Here's how the part is built. I have some questions about the finished solid (model axes, mm). Face numbers are marked on the shaded views. A direction names the side the tool comes from. Coordinates: 2 decimals unless noted, no trailing zeros. Order: outer loops, then holes, each group sorted by start corner. A loop starts at its lowest first (then second) coordinate and runs counter-clockwise, first axis right, second up. Notation, with made-up numbers: (12, 71) - (63, 71) arc R28 ccw to (63, 94) - close; hole circle Ø11 at (28, 27.25). An arc over 180 degrees is marked (long way). Answer in a Markdown table with one row per item. Add a question column.
Item 1: Will these pins go through, and if not, where does the flat tip stop? pin 1 Ø1 at (x, z) = (1, 1) entering from +Y; pin 2 Ø12 at (x, y) = (0, 0) entering from -Z; pin 3 Ø1.5 at (x, z) = (13, 4.5) entering from -Y; pin 4 Ø3 at (x, z) = (12.5, 4) entering from +Y.
Item 2: If I drill on line 1 along Y through (x, z) = (0, 3.5); line 2 along X through (y, z) = (-31, 0.5); line 3 along Y through (x, z) = (-35, 4.2), over which ranges is the centre line in solid material (lowest first)? Write a range as from..to.
Item 3: I want a section at C-C (x = -27.5). Please give me the cut outline in (y, z), plus the area to 3 significant figures.
Item 4: I want a section at A-A (x = 0). Please give me the cut outline in (y, z), plus the area to 3 significant figures.
Item 5: Thinking about a two-plate mould opening in Y: for the marked faces 1, 2, 3 and 4, which applies, +Y half, -Y half, draft (parallel to the pull), parting line (faces both ways), or undercut?
Item 6: I want a section at D-D (y = 12). Please give me the cut outline in (x, z).
Item 7: On a 3-axis mill with a long thin cutter (end or side, diameter ignored), from which of +Z, -Z, +X, -X, +Y, -Y can I reach the whole of each face in a straight line? I mean the marked faces 5, 6, 7 and 8. Say none if no direction works.
```python
from build123d import *

# Parameters (mm, degrees)
SKETCH1_R           = 40
SKETCH1_R_2         = 10
BOSS_EXTRUDE1_DEPTH = 6
CUT_EXTRUDE1_START  = -6
CUT_EXTRUDE1_DEPTH  = 6
CIRPATTERN1_DEPTH   = 6


# Read off the part's stored shape, not the designer's step: CirPattern1
with BuildPart() as part:
    # Sketch1 → Boss-Extrude1 (new body)
    with BuildSketch(Plane.XY):
        Circle(SKETCH1_R)
        Circle(SKETCH1_R_2, mode=Mode.SUBTRACT)
    extrude(amount=BOSS_EXTRUDE1_DEPTH)

    # Sketch2 → Cut-Extrude1 (cut)
    with BuildSketch(Plane.XY.offset(6).offset(CUT_EXTRUDE1_START)):
        with BuildLine():
            Line((-3.601715358, 39.837515566), (-1.869030862, 35.288154767))
            ThreePointArc((-1.869030862, 35.288154767), (0, 34), (1.869030862, 35.288154767))
            Line((1.869030862, 35.288154767), (3.601715358, 39.837515566))
            ThreePointArc((3.601715358, 39.837515566), (0, 40), (-3.601715358, 39.837515566))
        make_face()
    extrude(amount=CUT_EXTRUDE1_DEPTH, mode=Mode.SUBTRACT)

    # CirPattern1 outline → CirPattern1 (cut)
    with BuildSketch(Plane.XY):
        with BuildLine():
            Line((-13.789697621, 37.547892611), (-10.9385917, 33.601999269))
            ThreePointArc((-10.9385917, 33.601999269), (-8.799847533, 32.841478094), (-7.32790134, 34.569480835))
            Line((-7.32790134, 34.569480835), (-6.831717855, 39.41227767))
            ThreePointArc((-6.831717855, 39.41227767), (-10.352761804, 38.637033051), (-13.789697621, 37.547892611))
        make_face()
        with BuildLine():
            Line((10.9385917, 33.601999269), (13.789697621, 37.547892611))
            ThreePointArc((13.789697621, 37.547892611), (10.352761804, 38.637033051), (6.831717855, 39.41227767))
            Line((6.831717855, 39.41227767), (7.32790134, 34.569480835))
            ThreePointArc((7.32790134, 34.569480835), (8.799847533, 32.841478094), (10.9385917, 33.601999269))
        make_face()
        with BuildLine():
            Line((19.262705591, 29.62592305), (23.03793478, 32.699442825))
            ThreePointArc((23.03793478, 32.699442825), (20, 34.641016151), (16.799580786, 36.301158183))
            Line((16.799580786, 36.301158183), (16.025449176, 31.494953912))
            ThreePointArc((16.025449176, 31.494953912), (17, 29.444863729), (19.262705591, 29.62592305))
        make_face()
        with BuildLine():
            Line((26.274097929, 23.630889134), (30.716174756, 25.622580049))
            ThreePointArc((30.716174756, 25.622580049), (28.284271247, 28.284271247), (25.622580049, 30.716174756))
            Line((25.622580049, 30.716174756), (23.630889134, 26.274097929))
            ThreePointArc((23.630889134, 26.274097929), (24.04163056, 24.04163056), (26.274097929, 23.630889134))
        make_face()
        with BuildLine():
            Line((31.494953912, 16.025449176), (36.301158183, 16.799580786))
            ThreePointArc((36.301158183, 16.799580786), (34.641016151, 20), (32.699442825, 23.03793478))
            Line((32.699442825, 23.03793478), (29.62592305, 19.262705591))
            ThreePointArc((29.62592305, 19.262705591), (29.444863729, 17), (31.494953912, 16.025449176))
        make_face()
        with BuildLine():
            Line((34.569480835, 7.32790134), (39.41227767, 6.831717855))
            ThreePointArc((39.41227767, 6.831717855), (38.637033052, 10.352761804), (37.547892611, 13.789697621))
            Line((37.547892611, 13.789697621), (33.601999269, 10.9385917))
            ThreePointArc((33.601999269, 10.9385917), (32.841478094, 8.799847533), (34.569480835, 7.32790134))
        make_face()
        with BuildLine():
            Line((35.288154767, -1.869030862), (39.837515566, -3.601715358))
            ThreePointArc((39.837515566, -3.601715358), (40, 0), (39.837515566, 3.601715358))
            Line((39.837515566, 3.601715358), (35.288154767, 1.869030862))
            ThreePointArc((35.288154767, 1.869030862), (34, 0), (35.288154767, -1.869030862))
        make_face()
        with BuildLine():
            Line((33.601999269, -10.9385917), (37.547892611, -13.789697621))
            ThreePointArc((37.547892611, -13.789697621), (38.637033052, -10.352761804), (39.41227767, -6.831717855))
            Line((39.41227767, -6.831717855), (34.569480835, -7.32790134))
            ThreePointArc((34.569480835, -7.32790134), (32.841478094, -8.799847533), (33.601999269, -10.9385917))
        make_face()
        with BuildLine():
            Line((29.62592305, -19.262705591), (32.699442825, -23.03793478))
            ThreePointArc((32.699442825, -23.03793478), (34.641016151, -20), (36.301158183, -16.799580786))
            Line((36.301158183, -16.799580786), (31.494953912, -16.025449176))
            ThreePointArc((31.494953912, -16.025449176), (29.444863729, -17), (29.62592305, -19.262705591))
        make_face()
        with BuildLine():
            Line((23.630889134, -26.274097929), (25.622580049, -30.716174756))
            ThreePointArc((25.622580049, -30.716174756), (28.284271247, -28.284271247), (30.716174756, -25.622580049))
            Line((30.716174756, -25.622580049), (26.274097929, -23.630889134))
            ThreePointArc((26.274097929, -23.630889134), (24.04163056, -24.04163056), (23.630889134, -26.274097929))
        make_face()
        with BuildLine():
            Line((16.025449176, -31.494953912), (16.799580786, -36.301158183))
            ThreePointArc((16.799580786, -36.301158183), (20, -34.641016151), (23.03793478, -32.699442825))
            Line((23.03793478, -32.699442825), (19.262705591, -29.62592305))
            ThreePointArc((19.262705591, -29.62592305), (17, -29.444863729), (16.025449176, -31.494953912))
        make_face()
        with BuildLine():
            Line((7.32790134, -34.569480835), (6.831717855, -39.41227767))
            ThreePointArc((6.831717855, -39.41227767), (10.352761804, -38.637033052), (13.789697621, -37.547892611))
            Line((13.789697621, -37.547892611), (10.9385917, -33.601999269))
            ThreePointArc((10.9385917, -33.601999269), (8.799847533, -32.841478094), (7.32790134, -34.569480835))
        make_face()
        with BuildLine():
            Line((-1.869030862, -35.288154767), (-3.601715358, -39.837515566))
            ThreePointArc((-3.601715358, -39.837515566), (0, -40), (3.601715358, -39.837515566))
            Line((3.601715358, -39.837515566), (1.869030862, -35.288154767))
            ThreePointArc((1.869030862, -35.288154767), (0, -34), (-1.869030862, -35.288154767))
        make_face()
        with BuildLine():
            Line((-10.9385917, -33.601999269), (-13.789697621, -37.547892611))
            ThreePointArc((-13.789697621, -37.547892611), (-10.352761804, -38.637033052), (-6.831717855, -39.41227767))
            Line((-6.831717855, -39.41227767), (-7.32790134, -34.569480835))
            ThreePointArc((-7.32790134, -34.569480835), (-8.799847533, -32.841478094), (-10.9385917, -33.601999269))
        make_face()
        with BuildLine():
            Line((-19.262705591, -29.62592305), (-23.03793478, -32.699442825))
            ThreePointArc((-23.03793478, -32.699442825), (-20, -34.641016151), (-16.799580786, -36.301158183))
            Line((-16.799580786, -36.301158183), (-16.025449176, -31.494953912))
            ThreePointArc((-16.025449176, -31.494953912), (-17, -29.444863729), (-19.262705591, -29.62592305))
        make_face()
        with BuildLine():
            Line((-26.274097929, -23.630889134), (-30.716174756, -25.622580049))
            ThreePointArc((-30.716174756, -25.622580049), (-28.284271247, -28.284271247), (-25.622580049, -30.716174756))
            Line((-25.622580049, -30.716174756), (-23.630889134, -26.274097929))
            ThreePointArc((-23.630889134, -26.274097929), (-24.04163056, -24.04163056), (-26.274097929, -23.630889134))
        make_face()
        with BuildLine():
            Line((-31.494953912, -16.025449176), (-36.301158183, -16.799580786))
            ThreePointArc((-36.301158183, -16.799580786), (-34.641016151, -20), (-32.699442825, -23.03793478))
            Line((-32.699442825, -23.03793478), (-29.62592305, -19.262705591))
            ThreePointArc((-29.62592305, -19.262705591), (-29.444863729, -17), (-31.494953912, -16.025449176))
        make_face()
        with BuildLine():
            Line((-34.569480835, -7.32790134), (-39.41227767, -6.831717855))
            ThreePointArc((-39.41227767, -6.831717855), (-38.637033052, -10.352761804), (-37.547892611, -13.789697621))
            Line((-37.547892611, -13.789697621), (-33.601999269, -10.9385917))
            ThreePointArc((-33.601999269, -10.9385917), (-32.841478094, -8.799847533), (-34.569480835, -7.32790134))
        make_face()
        with BuildLine():
            Line((-35.288154767, 1.869030862), (-39.837515566, 3.601715358))
            ThreePointArc((-39.837515566, 3.601715358), (-40, 0), (-39.837515566, -3.601715358))
            Line((-39.837515566, -3.601715358), (-35.288154767, -1.869030862))
            ThreePointArc((-35.288154767, -1.869030862), (-34, 0), (-35.288154767, 1.869030862))
        make_face()
        with BuildLine():
            Line((-33.601999269, 10.9385917), (-37.547892611, 13.789697621))
            ThreePointArc((-37.547892611, 13.789697621), (-38.637033052, 10.352761804), (-39.41227767, 6.831717855))
            Line((-39.41227767, 6.831717855), (-34.569480835, 7.32790134))
            ThreePointArc((-34.569480835, 7.32790134), (-32.841478094, 8.799847533), (-33.601999269, 10.9385917))
        make_face()
        with BuildLine():
            Line((-29.62592305, 19.262705591), (-32.699442825, 23.03793478))
            ThreePointArc((-32.699442825, 23.03793478), (-34.641016151, 20), (-36.301158183, 16.799580786))
            Line((-36.301158183, 16.799580786), (-31.494953912, 16.025449176))
            ThreePointArc((-31.494953912, 16.025449176), (-29.444863729, 17), (-29.62592305, 19.262705591))
        make_face()
        with BuildLine():
            Line((-23.630889134, 26.274097929), (-25.622580049, 30.716174756))
            ThreePointArc((-25.622580049, 30.716174756), (-28.284271247, 28.284271247), (-30.716174756, 25.622580049))
            Line((-30.716174756, 25.622580049), (-26.274097929, 23.630889134))
            ThreePointArc((-26.274097929, 23.630889134), (-24.04163056, 24.04163056), (-23.630889134, 26.274097929))
        make_face()
        with BuildLine():
            Line((-16.025449176, 31.494953912), (-16.799580786, 36.301158183))
            ThreePointArc((-16.799580786, 36.301158183), (-20, 34.641016151), (-23.03793478, 32.699442825))
            Line((-23.03793478, 32.699442825), (-19.262705591, 29.62592305))
            ThreePointArc((-19.262705591, 29.62592305), (-17, 29.444863729), (-16.025449176, 31.494953912))
        make_face()
    extrude(amount=CIRPATTERN1_DEPTH, mode=Mode.SUBTRACT)


solid = part.part
```
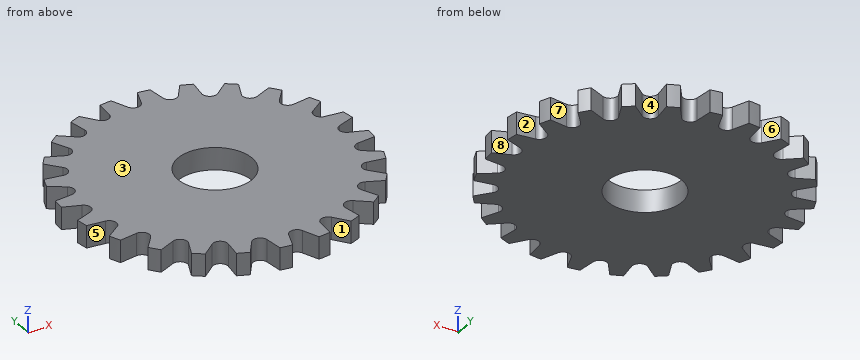
Values follow:
| question | item | result |
|---|---|---|
| 1 | pin 1 | stops at y = 34.68 |
| 1 | pin 2 | passes through |
| 1 | pin 3 | stops at y = -37.49 |
| 1 | pin 4 | stops at y = 37.55 |
| 2 | line 1 | y = -34..-10, 10..34 |
| 2 | line 2 | x = -25.28..-20.95, -16.01..16.01, 20.95..25.28 |
| 2 | line 3 | y = -16.59..-11.95, -7.28..-1.73, 1.73..7.28, 11.95..16.59 |
| 3 | outline | (-24.18, 0) - (24.18, 0) - (24.18, 6) - (-24.18, 6) - close |
| 3 | area | 290 mm^2 |
| 4 | outline | (-34, 0) - (-10, 0) - (-10, 6) - (-34, 6) - close; (10, 0) - (34, 0) - (34, 6) - (10, 6) - close |
| 4 | area | 288 mm^2 |
| 5 | face 1 | -Y half |
| 5 | face 2 | undercut |
| 5 | face 3 | draft |
| 5 | face 4 | undercut |
| 6 | outline | (-35.07, 0) - (35.07, 0) - (35.07, 6) - (-35.07, 6) - close |
| 7 | face 5 | +Z, -Z, -X |
| 7 | face 6 | +Z, -Z, +Y |
| 7 | face 7 | +Z, -Z |
| 7 | face 8 | +Z, -Z, +X |
